Answer from the drawing. Dimensions are ordinates in mm from the lowest x, y and z of the part. A direction names the side the tool comes from. Coordinates: 2 decimals unless noted, no trailing zeros. Write each loop counter-clockwise with the first axis right and the second up, starting at its lowest first coordinate (ties: lowest second). Pieces come first, ordered by that corner, then holes. Notation, with made-up numbers: (0.5, 69.25) - (32.5, 69.25) arc R15 cw to (32.5, 80.25) - close; hole circle Ø7 at (0.25, 45). An arc over 180 degrees is marked (long way). Return JSON: item names as keys, results as strings.
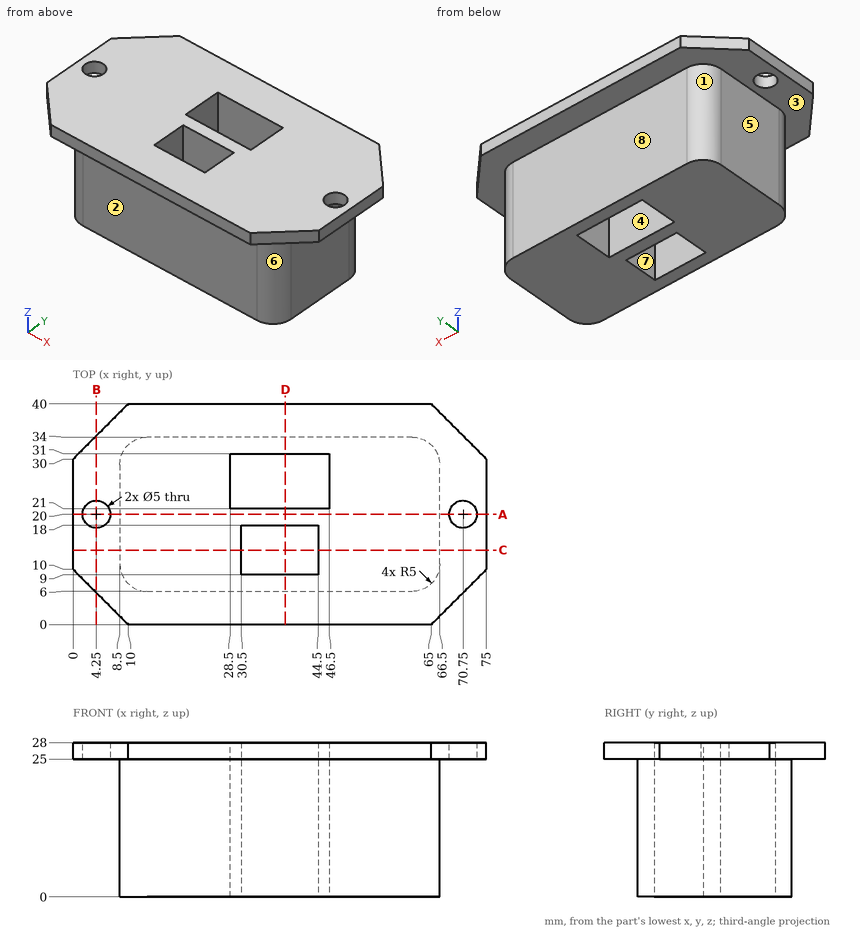
(1) Determine the mould class of the marked faces 5, 6, 7 and 8 for opening direction Y: +Y half, -Y half, draft (parallel to the pull), parting line (faces both ways), or undercut.
Answer:
{"face 5": "draft", "face 6": "-Y half", "face 7": "undercut", "face 8": "+Y half"}
(2) Straight lines are drawn through the part: line 1 (Y direction, x = 35, z = 9.5); line 2 (X direction, y = 11.5, z = 6.5); line 3 (Z direction, x = 67, y = 8). For each, find the intervals that lie inside material, in ascending order. Write a range as from..to.
Answer:
{"line 1": "6..9, 18..21, 31..34", "line 2": "8.5..30.5, 44.5..66.5", "line 3": "25..28"}
(3) A cutting plane is placed at A-A (y = 20). Determine the outline of the cut face in (x, z).
Answer:
{"outline": "(0, 25) - (1.75, 25) - (1.75, 28) - (0, 28) - close; (6.75, 25) - (8.5, 25) - (8.5, 0) - (66.5, 0) - (66.5, 25) - (68.25, 25) - (68.25, 28) - (6.75, 28) - close; (73.25, 25) - (75, 25) - (75, 28) - (73.25, 28) - close"}
(4) A cutting plane is placed at B-B (x = 4.25). Determine the outline of the cut face in (y, z), and give its area (3 significant figures).
Answer:
{"outline": "(5.75, 25) - (17.5, 25) - (17.5, 28) - (5.75, 28) - close; (22.5, 25) - (34.25, 25) - (34.25, 28) - (22.5, 28) - close", "area": "70.5 mm²"}
(5) Which of the six approach directions +Z, -Z, +X, -X, +Y, -Y give full straight-line access (tool end or side, diameter ignored) to the marked faces 1, 2, 3 and 4?
Answer:
{"face 1": "-Z, -X, +Y", "face 2": "-Z, +X, -X, -Y", "face 3": "-Z", "face 4": "+Z, -Z"}
(6) A cutting plane is placed at D-D (x = 38.5). Determine the outline of the cut face in (y, z), and give its area (3 significant figures).
Answer:
{"outline": "(0, 25) - (6, 25) - (6, 0) - (9, 0) - (9, 28) - (0, 28) - close; (18, 0) - (21, 0) - (21, 28) - (18, 28) - close; (31, 0) - (34, 0) - (34, 25) - (40, 25) - (40, 28) - (31, 28) - close", "area": "288 mm²"}
(7) Flat-ended cylindrical pins translate along their axes: P1, Ø3, axis at x = 13.5, z = 4.5, coming from the -Y side; P2, Ø14.5, axis at y = 16, z = 8, coming from the -X side; P3, Ø8, axis at x = 4.25, y = 20, coming from the -Z side. Find the tip coordinate at first contact, or state that the pin passes through.
Answer:
{"P1": "y = 6", "P2": "x = 8.5", "P3": "z = 25"}
(8) A cutting plane is placed at C-C (y = 13.5). Determine the outline of the cut face in (x, z).
Answer:
{"outline": "(0, 25) - (8.5, 25) - (8.5, 0) - (30.5, 0) - (30.5, 28) - (0, 28) - close; (44.5, 0) - (66.5, 0) - (66.5, 25) - (75, 25) - (75, 28) - (44.5, 28) - close"}
